from build123d import *

# Parameters (mm, degrees)
F1_DEPTH = 260
F2_SIZE  = 1


with BuildPart() as f1:
    # F0 (on Front) → F1 (new body)
    with BuildSketch(Plane.XZ):
        Polygon((0, 260), (0, 0), (1200, 0), (890.144066, 260), align=None)
        Polygon((22, 22), (22, 238), (882.136721, 238), (1139.555497, 22), align=None, mode=Mode.SUBTRACT)
    extrude(amount=F1_DEPTH)

    # F2
    f2_edges = [f1.edges().sort_by_distance(p)[0] for p in [
        (445.072033, -260, 260),
        (452.06836, -260, 238),
        (580.777748, -260, 22),
        (600, -260, 0),
        (0, -260, 130),
        (22, -260, 130),
        (1045.072033, -260, 130),
        (1010.846109, -260, 130),
        (580.777748, 0, 22),
        (445.072033, 0, 260),
        (1045.072033, 0, 130),
        (1010.846109, 0, 130),
        (452.06836, 0, 238),
        (0, 0, 130),
        (22, 0, 130),
        (600, 0, 0),
    ]]
    chamfer(f2_edges, length=F2_SIZE)


solid = f1.part
The listing builds one solid part. Answer for the finished solid, in the listing's coordinates (mm). A direction names the side the tool comes from. Give positions to 0.01 mm unless a question says otherwise; leave off trailing zeros. Write each loop counter-clockwise with the first axis right and the second up, starting at its lowest first coordinate (ties: lowest second). Pieces come first, ordered by that corner, then holes.
Item 1: Find the intervals of material crossed by line 1 along Z through (x, y) = (271, -60); line 2 along X through (y, z) = (-65, 48.5); line 3 along X through (y, z) = (-49.5, 34), in increasing order.
Item 2: Section B-B, the plane z = 55 is taken. Write down the section's boundary in (x, y).
Item 3: Flat-ended cylindrical pins translate along their axes: P1, Ø5, axis at x = 934.5, y = -76.5, coming from the +Z side; P2, Ø1.5, axis at x = 1011, y = -57.5, coming from the +Z side. Find the tip coordinate at first contact, or state that the pin passes through.
Item 4: Determine the mould class of faces 1 (the flat face through (1046.915, -259.507, 127.792)), 2 (the flat face through (508, -260, 16)), 3 (the flat face through (1010.27, -0.49, 131.15)) for opening direction X: released by +X, released by -X, zero draft, split by the parting line, or undercut.
Item 5: Section A-A, the plane x = 789 is taken. Write down the section's boundary in (y, z).
Item 6: Which of the six approach directions +Z, -Z, +X, -X, +Y, -Y give full straight-line access (tool end or side, diameter ignored) to faces 4 (the flat face through (1047.24, -128.19, 128.18)), 5 (the flat face through (446, -128, 238)), 6 (the flat face through (1010.27, -259.51, 131.15))?
Item 7: Section C-C, the plane y = -151 is taken. Write down the section's boundary in (x, z).
Completed:
1. line 1: z = 0 to 22, 238 to 260
1. line 2: x = 0 to 22, 1107.97 to 1142.2
1. line 3: x = 0 to 22, 1125.25 to 1159.48
2. outline: (0, -259) - (1, -260) - (21, -260) - (22, -259) - (22, -1) - (21, 0) - (1, 0) - (0, -1) - close; (1100.23, -259) - (1101.78, -260) - (1132.9, -260) - (1134.45, -259) - (1134.45, -1) - (1132.9, 0) - (1101.78, 0) - (1100.23, -1) - close
3. P1: stops at z = 224.88
3. P2: stops at z = 159.22
4. face 1: released by +X
4. face 2: zero draft
4. face 3: undercut
5. outline: (-260, 1) - (-259, 0) - (-1, 0) - (0, 1) - (0, 21) - (-1, 22) - (-259, 22) - (-260, 21) - close; (-260, 239) - (-259, 238) - (-1, 238) - (0, 239) - (0, 259) - (-1, 260) - (-259, 260) - (-260, 259) - close
6. face 4: +Z, +X, +Y, -Y
6. face 5: +Y, -Y
6. face 6: -Y
7. outline: (0, 0) - (1200, 0) - (890.14, 260) - (0, 260) - close; hole (22, 22) - (1139.56, 22) - (882.14, 238) - (22, 238) - close
